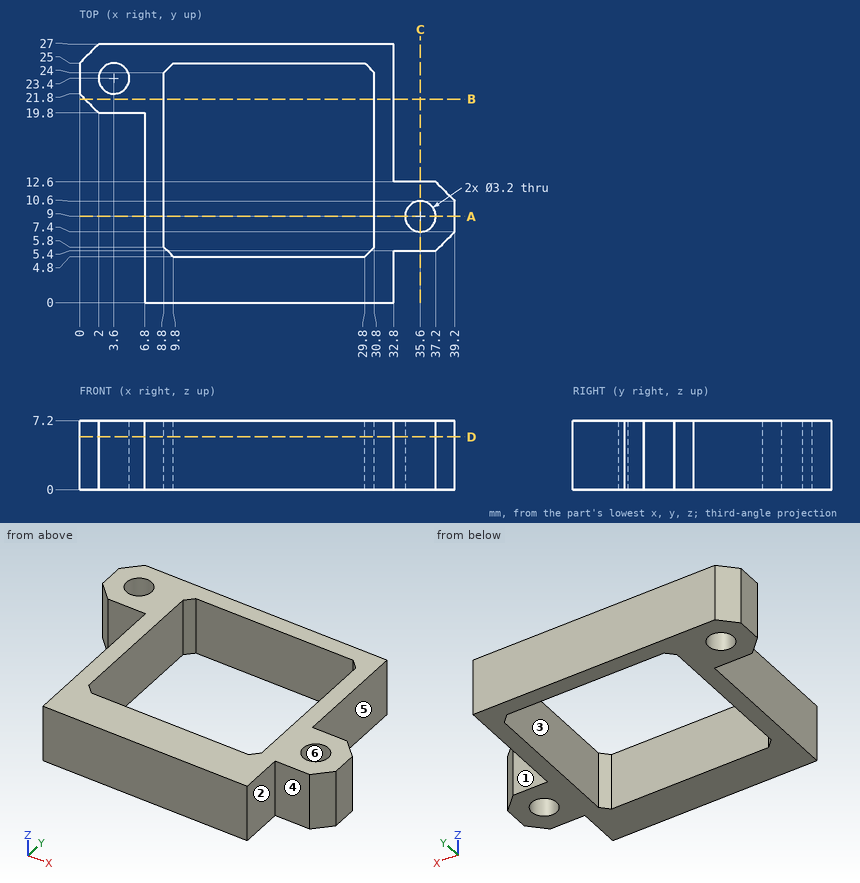
Geometry check sheet. Reference: drawing and pictorial views, mm from the part's lowest x, y, z. A direction names the side the tool comes from. Round coordinates to 2 decimals unless told otherwise and drop trailing zeros. Loops run counter-clockwise (first coordinate to the right, second up) from the corner with the lowest first, then second, coordinate; pieces in that order, holes last. Notation, with made-up numbers: (1.25, 72) - (44.25, 72) arc R30 cw to (44.25, 108) - close; hole circle Ø3 at (86.5, 65.5). An arc over 180 degrees is marked (long way). Answer in a Markdown table with one row per item. Add a question column.
Q1. Section check B-B on y = 21.25. Enter the section's corners in (x, z).
Q2. Material ranges on line 1 (Y direction, x = 17, z = 4.5); line 2 (X direction, y = 12.75, z = 5.5); line 3 (Y direction, x = 3.6, z = 1.5), recorded low to high.
Q3. Section check C-C on x = 35.6. Enter the section's corners in (y, z).
Q4. Release check for a two-part mould opening along Y. For the marked faces 4, 5 and 6 record: pulls with the +Y half, pulls with the -Y half, needs draft (parallel to the pull), parting line crosses it, or undercut.
Q5. Tool access check on the marked faces 1, 2 and 3. Record the directions out of +Z, -Z, +X, -X, +Y, -Y that give a thin tool (end or side, any length) a straight path to the whole face; none if there is none.
Q6. Gauge pin test, flat ends, axial feed: pin 1 (1.6 mm diameter, centred on y = 3, z = 5, fed in from +X); pin 2 (1.5 mm diameter, centred on y = 6.5, z = 5.5, fed in from -X); pin 3 (1.3 mm diameter, centred on x = 36, z = 4, fed in from -Y). Record the tip position at first contact, or that the pin passes through.
Q7. Section check A-A on y = 9. Enter the section's corners in (x, z), plus the area to 3 significant figures.
Q8. Section check D-D on z = 5.5. Enter the section's corners in (x, y).
Found:
| question | item | result |
|---|---|---|
| 1 | outline | (0.55, 0) - (8.8, 0) - (8.8, 7.2) - (0.55, 7.2) - close; (30.8, 0) - (32.8, 0) - (32.8, 7.2) - (30.8, 7.2) - close |
| 2 | line 1 | y = 0 to 4.8, 25 to 27 |
| 2 | line 2 | x = 6.8 to 8.8, 30.8 to 32.8 |
| 2 | line 3 | y = 19.8 to 21.8, 25 to 27 |
| 3 | outline | (5.4, 0) - (7.4, 0) - (7.4, 7.2) - (5.4, 7.2) - close; (10.6, 0) - (12.6, 0) - (12.6, 7.2) - (10.6, 7.2) - close |
| 4 | face 4 | pulls with the -Y half |
| 4 | face 5 | needs draft |
| 4 | face 6 | undercut |
| 5 | face 1 | +Z, -Z, +X, +Y |
| 5 | face 2 | +Z, -Z, +X, -Y |
| 5 | face 3 | +Z, -Z |
| 6 | pin 1 | stops at x = 32.8 |
| 6 | pin 2 | stops at x = 6.8 |
| 6 | pin 3 | stops at y = 5.4 |
| 7 | outline | (6.8, 0) - (8.8, 0) - (8.8, 7.2) - (6.8, 7.2) - close; (30.8, 0) - (34, 0) - (34, 7.2) - (30.8, 7.2) - close; (37.2, 0) - (39.2, 0) - (39.2, 7.2) - (37.2, 7.2) - close |
| 7 | area | 51.8 mm² |
| 8 | outline | (0, 21.8) - (2, 19.8) - (6.8, 19.8) - (6.8, 0) - (32.8, 0) - (32.8, 5.4) - (37.2, 5.4) - (39.2, 7.4) - (39.2, 10.6) - (37.2, 12.6) - (32.8, 12.6) - (32.8, 27) - (2, 27) - (0, 25) - close; hole circle Ø3.2 at (3.6, 23.4); hole (8.8, 5.8) - (9.8, 4.8) - (29.8, 4.8) - (30.8, 5.8) - (30.8, 24) - (29.8, 25) - (9.8, 25) - (8.8, 24) - close; hole circle Ø3.2 at (35.6, 9) |
